```python
from build123d import *

# Parameters (mm, degrees)
SKETCH3_W           = 93.98
SKETCH3_H           = 50.8
BOSS_EXTRUDE1_DEPTH = 27.94
SKETCH4_W           = 72.39
SKETCH4_H           = 50.8
CUT_EXTRUDE1_DEPTH  = 27.94
FILLET1_R           = 22.86
SKETCH5_W           = 21.59
SKETCH5_H           = 10.16
BOSS_EXTRUDE2_DEPTH = 2.54
FILLET2_R           = 2.54
SKETCH6_R           = 2.249999945
CUT_EXTRUDE2_DEPTH  = 2.54
SKETCH7_W           = 3.81
SKETCH7_H           = 2.286
CUT_EXTRUDE3_DEPTH  = 7.62
SKETCH8_R           = 15.621
CUT_EXTRUDE4_DEPTH  = 15.24
FILLET3_R           = 27.94


# Read off the part's stored shape, not the designer's step: Cavity1
with BuildPart() as part:
    # Sketch3 → Boss-Extrude1 (new body)
    with BuildSketch(Plane.XY):
        with Locations((-42.520322955, 0)):
            Rectangle(SKETCH3_W, SKETCH3_H)
    extrude(amount=BOSS_EXTRUDE1_DEPTH)

    # Cavity1 outline → Cavity1 (revolve, cut)
    with BuildSketch(Plane.YX):
        with BuildLine():
            Line((0, -89.510322955), (14.536498149, -89.510322955))
            Line((14.536498149, -89.510322955), (17.81175, -66.58356))
            Line((17.81175, -66.58356), (6.477, -66.58356))
            Line((6.477, -66.58356), (6.477, -17.35836))
            Line((6.477, -17.35836), (23.05812, -17.35836))
            ThreePointArc((23.05812, -17.35836), (21.288451872, -10.075162449), (18.689240956, -3.045169955))
            ThreePointArc((18.689240956, -3.045169955), (17.939550019, -2.064315438), (16.821043187, -1.541769218))
            ThreePointArc((16.821043187, -1.541769218), (11.026301594, -0.582300423), (5.1816, 0))
            Line((5.1816, 0), (4.864997876, 4.469677045))
            Line((4.864997876, 4.469677045), (0, 4.469677045))
            Line((0, 4.469677045), (0, -89.510322955))
        make_face()
    revolve(axis=Axis((0, 0, 0), (1, 0, 0)), mode=Mode.SUBTRACT)

    # Sketch4 → Cut-Extrude1 (cut)
    with BuildSketch(Plane(origin=(0, 0, 0), x_dir=(-1, 0, 0), z_dir=(0, 0, -1))):
        with Locations((31.725322955, 0)):
            Rectangle(SKETCH4_W, SKETCH4_H)
    extrude(amount=-CUT_EXTRUDE1_DEPTH, mode=Mode.SUBTRACT)

    # Fillet1
    fillet1_edges = [part.edges().sort_by_distance(p)[0] for p in [
        (-78.715322955, 25.4, 27.94),
        (-78.715322955, -25.4, 27.94),
    ]]
    fillet(fillet1_edges, radius=FILLET1_R)

    # Sketch5 → Boss-Extrude2 (add)
    with BuildSketch(Plane(origin=(0, 0, 0), x_dir=(-1, 0, 0), z_dir=(0, 0, -1))):
        with Locations((78.715322955, 30.48)):
            Rectangle(SKETCH5_W, SKETCH5_H)
        with Locations((78.715322955, -30.48)):
            Rectangle(SKETCH5_W, SKETCH5_H)
    extrude(amount=-BOSS_EXTRUDE2_DEPTH)

    # Fillet2
    fillet2_edges = [part.edges().sort_by_distance(p)[0] for p in [
        (-89.510322955, 35.56, 1.27),
        (-67.920322955, 35.56, 1.27),
        (-89.510322955, -35.56, 1.27),
        (-67.920322955, -35.56, 1.27),
    ]]
    fillet(fillet2_edges, radius=FILLET2_R)

    # Sketch6 → Cut-Extrude2 (cut)
    with BuildSketch(Plane.XY.offset(2.54)):
        with Locations((-84.430322955, 30.48)):
            Circle(SKETCH6_R)
        with Locations((-73.000322955, 30.48)):
            Circle(SKETCH6_R)
        with Locations((-84.430322955, -30.48)):
            Circle(SKETCH6_R)
        with Locations((-73.000322955, -30.48)):
            Circle(SKETCH6_R)
    extrude(amount=-CUT_EXTRUDE2_DEPTH, mode=Mode.SUBTRACT)

    # Sketch7 → Cut-Extrude3 (cut)
    with BuildSketch(Plane(origin=(-67.920322955, 0, 0), x_dir=(0, 0, -1), z_dir=(1, 0, 0))):
        with Locations((-18.509783864, 0)):
            Rectangle(SKETCH7_W, SKETCH7_H)
    extrude(amount=-CUT_EXTRUDE3_DEPTH, mode=Mode.SUBTRACT)

    # Sketch8 → Cut-Extrude4 (cut)
    with BuildSketch(Plane.ZY.offset(89.510322955)):
        Circle(SKETCH8_R)
    extrude(amount=-CUT_EXTRUDE4_DEPTH, mode=Mode.SUBTRACT)

    # Fillet3
    fillet3_edges = [part.edges().sort_by_distance(p)[0] for p in [
        (-81.918809999, 0, 15.621),
    ]]
    fillet(fillet3_edges, radius=FILLET3_R)


solid = part.part
```
Design review of the part built by this model. Coordinates are the model's own, in mm. A direction names the side the tool comes from. Give positions to 0.01 mm unless a question says otherwise; leave off trailing zeros. Order: outer loops, then holes, each group sorted by start corner. A loop starts at its lowest first (then second) coordinate and runs counter-clockwise, first axis right, second up. Notation, with made-up numbers: (-15, 24.5) - (40, 24.5) arc R21 ccw to (40, 60.5) - close; hole circle Ø4 at (-2.75, 48.5). An arc over 180 degrees is marked (long way). Use a Markdown table: item, result. Add a question column.
(1) Wall thickness on probe 1 along Y at (x, z) = (-70.5, 1.75); probe 2 along Y at (x, z) = (-86, 2.75); probe 3 along Z at (x, y) = (-82.5, 32.5): over which ranges is each line inside the solid? List them lowest first. Write a range as [from, to].
(2) Machinability: for faces 4 (the face through (-67.92, 7, 17)), 5 (the face through (-79, 31, 2.54)), 6 (the face through (-72, 1.143, 19)), which of the approach directions +Z, -Z, +X, -X, +Y, -Y give a long, thin tool a straight path to every point of the face, cutting with its end or side? Answer none if there is none.
(3) Clearance check with flat-ended pins moving along their axes: P1, Ø3, axis at x = -70.5, z = 19, coming from the -Y side; P2, Ø2.5, axis at x = -73, y = -30.48, coming from the +Z side; P3, Ø8, axis at x = -82.5, y = -33, coming from the +Z side; P4, Ø1, axis at x = -77.5, z = 5.5, coming from the -Y side. State where each tip first meets the part, or that it passes through.
(4) Add section A-A on y = -30.48. Give the boundary of the cut face in (x, z), then the cut area to 3 significant figures.
(5) Mouldability with a two-part tool opening along Y and no side actions: class faces 1 (the face through (-88.786, -34.796, 1.288)), 2 (the face through (-79, 26, 0)), 3 (the face through (-71.791, -28.583, 1.288)) as +Y half, -Y half, draft (parallel to the pull), parting line (faces both ways), or undercut.
Report:
| question | item | result |
|---|---|---|
| 1 | probe 1 | y = [-35.56, -17.16], [17.16, 35.56] |
| 1 | probe 2 | y = [-25.4, -15.38], [15.38, 25.4] |
| 1 | probe 3 | z = [0, 2.54] |
| 2 | face 4 | +Z, -Z, +X, +Y, -Y |
| 2 | face 5 | +Z, +X, -X, +Y |
| 2 | face 6 | +X |
| 3 | P1 | stops at y = -21.73 |
| 3 | P2 | passes through |
| 3 | P3 | stops at z = 2.54 |
| 3 | P4 | stops at y = -25.4 |
| 4 | outline | (-89.51, 0) - (-86.68, 0) - (-86.68, 2.54) - (-89.51, 2.54) - close; (-82.18, 0) - (-75.25, 0) - (-75.25, 2.54) - (-82.18, 2.54) - close; (-70.75, 0) - (-67.92, 0) - (-67.92, 2.54) - (-70.75, 2.54) - close |
| 4 | area | 32.0 mm² |
| 5 | face 1 | -Y half |
| 5 | face 2 | draft |
| 5 | face 3 | undercut |
